Geometry check sheet. Reference: the model listing, model coordinates, mm. Coordinates: 2 decimals unless noted, no trailing zeros. Loops run counter-clockwise (first coordinate to the right, second up) from the corner with the lowest first, then second, coordinate; pieces in that order, holes last.
from build123d import *

# Parameters (mm, degrees)
F0_W     = 200
F0_H     = 98.15
F1_DEPTH = 20
F3_DEPTH = 200.001
F4_DEPTH = 200.001


with BuildPart() as f1:
    # F0 (on Top) → F1 (new body)
    with BuildSketch(Plane.XY):
        Rectangle(F0_W, F0_H)
    extrude(amount=F1_DEPTH)

    # F2 (on face) → F3 (cut, through all)
    with BuildSketch(Plane(origin=(-100, 0, 0), x_dir=(0, -1, 0), z_dir=(-1, 0, 0))):
        Polygon((-37.527995, 0), (-49.075, 20), (-49.075, 0), align=None)
        Polygon((37.527995, 20), (49.075, 0), (49.075, 20), align=None)
    extrude(amount=-F3_DEPTH, mode=Mode.SUBTRACT)

    # F2 (on face) → F4 (cut, through all)
    with BuildSketch(Plane(origin=(-100, 0, 0), x_dir=(0, -1, 0), z_dir=(-1, 0, 0))):
        Polygon((-37.527995, 0), (-49.075, 20), (-49.075, 0), align=None)
        Polygon((37.527995, 20), (49.075, 0), (49.075, 20), align=None)
    extrude(amount=-F4_DEPTH, mode=Mode.SUBTRACT)


solid = f1.part
1) Material ranges on probe 1 along Y at (x, z) = (-29.5, 2.5); probe 2 along Y at (x, z) = (-90.5, 14.5), recorded low to high.
Data:
probe 1: y = -47.63 to 38.97
probe 2: y = -40.7 to 45.9
2) Section check B-B on z = 5. Record the cut outline in (x, y).
Data:
outline: (-100, -46.19) - (100, -46.19) - (100, 40.41) - (-100, 40.41) - close
3) Depth check by flat-ended pin: pin 1 (3 mm diameter, centred on x = 37, z = 2, fed in from +Y); pin 2 (1.5 mm diameter, centred on x = -24, z = 11, fed in from -Y). Enter the tip coordinate at first touch or a pass-through.
Data:
pin 1: stops at y = 39.55
pin 2: stops at y = -43.16
4) Section check A-A on x = -6. Record the cut outline in (y, z) (3 decimals).
Data:
outline: (-49.075, 0) - (37.528, 0) - (49.075, 20) - (-37.528, 20) - close
